Geometry check sheet. Reference: the model listing, model coordinates, mm. Face numbers are marked on the shaded views. A direction names the side the tool comes from. Give positions to 0.01 mm unless a question says otherwise; leave off trailing zeros. Write each loop counter-clockwise with the first axis right and the second up, starting at its lowest first coordinate (ties: lowest second). Pieces come first, ordered by that corner, then holes. Notation, with made-up numbers: (83, 74) -> (111, 74) arc R30 cw to (111, 96) -> close; hole circle Ø8 at (63, -3). An arc over 180 degrees is marked (long way). One line per item, written item: value.
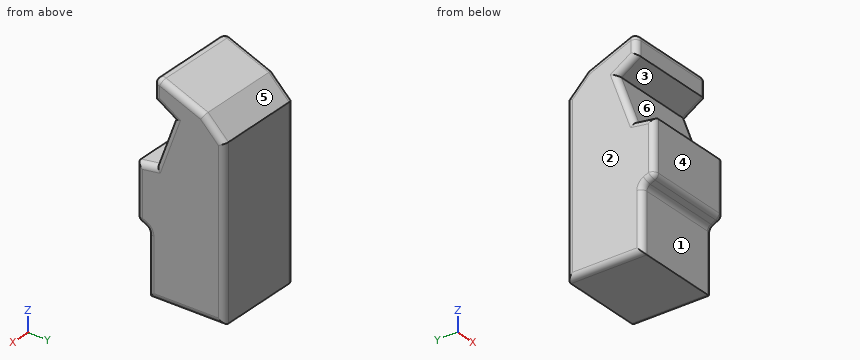
from build123d import *

# Parameters (mm, degrees)
F1_DEPTH = 39.652094
F2_R     = 5


with BuildPart() as f1:
    # F0 (on Right) → F1 (new body, symmetric)
    with BuildSketch(Plane.YZ):
        Polygon((-66, 0), (0, 0), (0, 145), (-17.67767, 162.67767), (-61, 180), (-61, 160), (-43.964932, 149.316322), (-59.184828, 107.5), (-76, 105), (-76, 58.582576), (-66, 54), align=None)
    extrude(amount=F1_DEPTH, both=True)

    # F2
    f2_edges = [f1.edges().sort_by_distance(p)[0] for p in [
        (0, -76, 58.582576),
        (0, -66, 54),
        (-39.652094, -66, 27),
        (-39.652094, -76, 81.791288),
        (-39.652094, -67.592414, 106.25),
        (-39.652094, -51.57488, 128.408161),
        (-39.652094, -33, 0),
        (-39.652094, 0, 72.5),
        (-39.652094, -8.838835, 153.838835),
        (-39.652094, -39.338835, 171.338835),
        (-39.652094, -61, 170),
        (-39.652094, -52.482466, 154.658161),
        (-39.652094, -71, 56.291288),
        (39.652094, -33, 0),
        (39.652094, 0, 72.5),
        (39.652094, -8.838835, 153.838835),
        (39.652094, -39.338835, 171.338835),
        (39.652094, -61, 170),
        (39.652094, -52.482466, 154.658161),
        (39.652094, -51.57488, 128.408161),
        (39.652094, -67.592414, 106.25),
        (39.652094, -76, 81.791288),
        (39.652094, -71, 56.291288),
        (39.652094, -66, 27),
        (0, -61, 180),
    ]]
    fillet(f2_edges, radius=F2_R)


solid = f1.part
1) Mould release check, pull along Z, two halves, no side actions. Record for the marked faces 3, 4, 5 and 6: released by +Z, released by -Z, zero draft, split by the parting line, or undercut.
Verdict:
face 3: undercut
face 4: zero draft
face 5: released by +Z
face 6: undercut
2) Sectioned sample at A-A on x = -28. Record the cut outline in (y, z).
Verdict:
outline: (-76, 61.79) arc R5 ccw to (-73.08, 57.25) -> (-68.92, 55.34) arc R5 cw to (-66, 50.79) -> (-66, 0) -> (0, 0) -> (0, 145) -> (-17.68, 162.68) -> (-54.14, 177.26) arc R5 ccw to (-61, 172.62) -> (-61, 160) -> (-43.96, 149.32) -> (-59.18, 107.5) -> (-76, 105) -> close
3) Scan lines: probe 1 along Y at (x, z) = (-25, 13.5); probe 2 along Z at (x, y) = (-22.5, -60); probe 3 along X at (y, z) = (-56.5, 165.5). Record each from-to range of solid material in increasing order.
Verdict:
probe 1: -66 to 0
probe 2: 0 to 107.38, 159.37 to 175.62
probe 3: -39.63 to 39.63
4) Depth check by flat-ended pin: pin 1 Ø5 at (x, y) = (-20, -63) entering from +Z; pin 2 Ø6 at (x, z) = (-8, 158.5) entering from +Y; pin 3 Ø5 at (x, z) = (-24, 141) entering from -Y. Enter the tip coordinate at first touch or a pass-through.
Verdict:
pin 1: z = 174.8
pin 2: y = -10.5
pin 3: y = -47.9
5) Tool access check on the marked faces 1 and 2. Record the directions out of +Z, -Z, +X, -X, +Y, -Y that give a thin tool (end or side, any length) a straight path to the whole face; none if there is none.
Verdict:
face 1: -Z, +X, -X, -Y
face 2: +Z, -Z, -X, +Y, -Y
